Check sheet for the modelled part. Datum: model origin and axes. Units: mm. Face numbers are marked on the shaded views. Round coordinates to 2 decimals unless told otherwise and drop trailing zeros. Write each loop counter-clockwise with the first axis right and the second up, starting at its lowest first coordinate (ties: lowest second). Pieces come first, ordered by that corner, then holes.
Item 1: Go/stop test with flat-tipped pins: pin 1 Ø2.5 at (x, y) = (0, 0) entering from -Z; pin 2 Ø4 at (x, z) = (-2, 25.5) entering from +Y; pin 3 Ø5 at (x, z) = (13.5, 18) entering from -Y. Record where each tip stops, or that it passes through.
Item 2: Cross-section at D-D on z = 6.5. Enter the section's corners in (x, y) (1 decimal), plus the area to 3 significant figures.
Item 3: Material ranges on line 1 (Y direction, x = 0, z = 58); line 2 (Y direction, x = 0, z = 15); line 3 (X direction, y = 0, z = 10.5), recorded low to high.
Item 4: Release check for a two-part mould opening along X. For the marked faces 1, 2 and 3 record: +X half, -X half, draft (parallel to the pull), parting line (faces both ways), or undercut.
Item 5: Cross-section at C-C on z = 42. Enter the section's corners in (x, y).
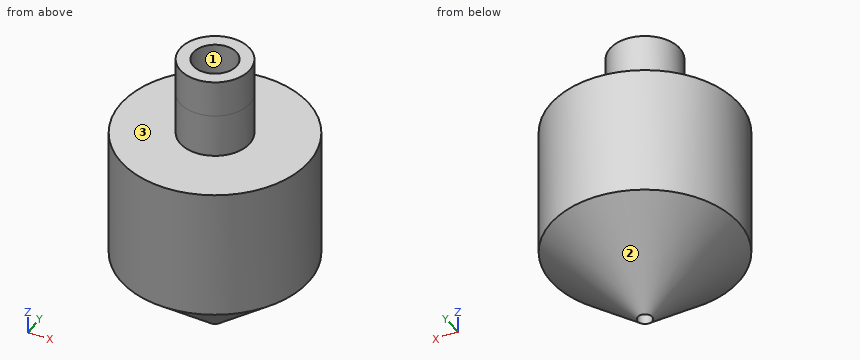
from build123d import *

# Parameters (mm, degrees)
F2_R         = 4.7625
F1_FACE1_R   = 20.5612294376
F1_FACE1_R_2 = 7.62
F3_DEPTH     = 9.525
F4_R         = 1.5875
F5_DEPTH     = 19.05


with BuildPart() as f1:
    # F0 (on Front) → F1 (revolve)
    with BuildSketch(Plane.XZ):
        Polygon((0, 63.5), (0, 0), (20.5612294376, 17.3543042779), (20.5612294376, 55.4543042779), (7.62, 55.4543042779), (7.62, 63.5), align=None)
    revolve(axis=Axis((0, 0, 31.75), (0, 0, -1)))

    # F2 (on face) + F1_face1 (on face) → F3 (cut)
    with BuildSketch(Plane.XY.offset(63.5)):
        Circle(F2_R)
    with BuildSketch(Plane.XY.offset(55.4543042779)):
        Circle(F1_FACE1_R)
        Circle(F1_FACE1_R_2, mode=Mode.SUBTRACT)
    extrude(amount=-F3_DEPTH, mode=Mode.SUBTRACT)

    # F4 (on Top) → F5 (cut)
    with BuildSketch(Plane.XY):
        Circle(F4_R)
    extrude(amount=F5_DEPTH, mode=Mode.SUBTRACT)


solid = f1.part
Response values:
1. pin 1: stops at z = 19.05
1. pin 2: stops at y = 20.56
1. pin 3: stops at y = -17.37
2. outline: circle Ø15.4 at (0, 0); hole circle Ø3.2 at (0, 0)
2. area: 178 mm2
3. line 1: y = -7.62 to -4.76, 4.76 to 7.62
3. line 2: y = -17.77 to -1.59, 1.59 to 17.77
3. line 3: x = -12.44 to -1.59, 1.59 to 12.44
4. face 1: undercut
4. face 2: parting line
4. face 3: draft
5. outline: circle Ø41.12 at (0, 0)
